from build123d import *

# Parameters (mm, degrees)
F0_R     = 39.206734
F0_R_2   = 3.455117
F0_R_3   = 3.683637
F0_R_4   = 20.926103
F0_R_5   = 3.503953
F0_R_6   = 3.247211
F1_DEPTH = 12.7
F2_DEPTH = 37.846
F3_R     = 11.90838
F4_DEPTH = 35.814


with BuildPart() as f1:
    # F0 (on Front) → F1 (new body)
    with BuildSketch(Plane.XZ):
        Circle(F0_R)
        with Locations((0, -31.248145)):
            Circle(F0_R_2, mode=Mode.SUBTRACT)
        with Locations((-31.432498, 0)):
            Circle(F0_R_3, mode=Mode.SUBTRACT)
        Circle(F0_R_4, mode=Mode.SUBTRACT)
        with Locations((31.432498, 0)):
            Circle(F0_R_5, mode=Mode.SUBTRACT)
        with Locations((0, 30.695081)):
            Circle(F0_R_6, mode=Mode.SUBTRACT)
    extrude(amount=F1_DEPTH)

    # F0 (on Front) → F2 (join)
    with BuildSketch(Plane.XZ):
        Circle(F0_R_4)
    extrude(amount=F2_DEPTH)

    # F3 (on face) → F4 (cut)
    with BuildSketch(Plane.XZ.offset(37.846)):
        Circle(F3_R)
    extrude(amount=-F4_DEPTH, mode=Mode.SUBTRACT)


solid = f1.part
Geometry: final body of the model. Coordinates: model frame, mm. A direction names the side the tool comes from. Give positions to 0.01 mm unless a question says otherwise; leave off trailing zeros. Loops run counter-clockwise (first coordinate to the right, second up) from the corner with the lowest first, then second, coordinate; pieces in that order, holes last. Notation, with made-up numbers: (4.25, 41) - (56.25, 41) arc R34 ccw to (56.25, 76) - close; hole circle Ø8 at (71.5, 76.25). An arc over 180 degrees is marked (long way). Answer as CSV lines item,"result". Start each with the question number.
1. Draft query along Z for faces 3 (the face through (-8.499, -6.261, -38.274)), 4 (the face through (9, -37.846, -9)), 5 (the face through (6.402, -20.19, 10.041)). Return one class per face: released by +Z, released by -Z, zero draft, split by the parting line, or undercut.
2. Section B-B, the plane x = 0. Return loops of the section in (y, z).
3. Section C-C, the plane y = -18. Return loops of the section in (x, z), plus the area to 3 significant figures.
4. Section D-D, the plane x = -10.5. Return loops of the section in (y, z).
5. Pin query (flat end, axial travel): P1, Ø6, axis at x = 0, z = 30.7, coming from the -Y side; P2, Ø11, axis at x = 31.43, z = 0, coming from the +Y side; P3, Ø1.5, axis at x = 4.5, y = -27, coming from the -Z side; P4, Ø8, axis at x = 8, y = -9, coming from the +Z side. Return the tip coordinate at first contact, or that it passes through.
6. Reachability of faces 1 (the face through (17, -12.7, -17)), 2 (the face through (-28.03, -6.26, -1.41)) from +Z, -Z, +X, -X, +Y, -Y: full face, straight path, thin tool, end or side. Return the list, or none.
7. Section A-A, the plane z = 0. Return loops of the section in (x, y), plus the area to 3 significant figures.
8. Ray query, L1, parallel to Z at x = 0, y = -9.5; L2, parallel to Y at x = 5.5, z = 4.5; L3, parallel to Y at x = 9.5, z = 36. Return the intervals inside material, ascending.
Answers:
1,face 3,"split by the parting line"
1,face 4,"zero draft"
1,face 5,"undercut"
2,outline,"(-37.85, -20.93) - (-12.7, -20.93) - (-12.7, -27.79) - (0, -27.79) - (0, 27.45) - (-12.7, 27.45) - (-12.7, 20.93) - (-37.85, 20.93) - (-37.85, 11.91) - (-2.03, 11.91) - (-2.03, -11.91) - (-37.85, -11.91) - close; (-12.7, -39.21) - (0, -39.21) - (0, -34.7) - (-12.7, -34.7) - close; (-12.7, 33.94) - (0, 33.94) - (0, 39.21) - (-12.7, 39.21) - close"
3,outline,"circle Ø41.85 at (0, 0); hole circle Ø23.82 at (0, 0)"
3,area,"930 mm2"
4,outline,"(-37.85, -18.1) - (-12.7, -18.1) - (-12.7, -37.77) - (0, -37.77) - (0, 37.77) - (-12.7, 37.77) - (-12.7, 18.1) - (-37.85, 18.1) - (-37.85, 5.62) - (-2.03, 5.62) - (-2.03, -5.62) - (-37.85, -5.62) - close"
5,P1,"passes through"
5,P2,"stops at y = 0"
5,P3,"stops at z = -20.59"
5,P4,"stops at z = 39"
6,face 1,"-Y"
6,face 2,"+Y, -Y"
7,outline,"(-39.21, -12.7) - (-35.12, -12.7) - (-35.12, 0) - (-39.21, 0) - close; (-27.75, -12.7) - (-20.93, -12.7) - (-20.93, -37.85) - (-11.91, -37.85) - (-11.91, -2.03) - (11.91, -2.03) - (11.91, -37.85) - (20.93, -37.85) - (20.93, -12.7) - (27.93, -12.7) - (27.93, 0) - (-27.75, 0) - close; (34.94, -12.7) - (39.21, -12.7) - (39.21, 0) - (34.94, 0) - close"
7,area,"1,010 mm2"
8,L1,"z = -39.21 to -34.7, -27.79 to -11.91, 11.91 to 27.45, 33.94 to 39.21"
8,L2,"y = -2.03 to 0"
8,L3,"y = -12.7 to 0"
